Source: three-view drawing plus pictorial views. Frame: mm from the lowest corner of the part. Give positions to 0.01 mm unless a question says otherwise; leave off trailing zeros. Loops run counter-clockwise (first coordinate to the right, second up) from the corner with the lowest first, then second, coordinate; pieces in that order, holes last. Notation, with made-up numbers: M -36.5,-36.5 L -26.5,-36.5 A22 ccw -26.5,-7.5 Z; hole C 9.5,84 d2. An arc over 180 degrees is marked long. Answer as a JSON object with one key per item and string values. Group by question number.
1) Section query D-D on y = 14.25. Return loops of the section in (x, z), plus the area to 3 significant figures.
2) Section query A-A on y = 9.3. Return loops of the section in (x, z).
3) First-contact query: P1, Ø1.5, axis at x = 12, z = 4.5, coming from the -Y side; P2, Ø6, axis at y = 12.5, z = 10.5, coming from the +X side; P3, Ø4, axis at x = 2, z = 12, coming from the -Y side. Flat tips, straight axial feed; report the tip coordinate or a pass-through.
4) Draft query along Y for the marked faces 1, 2 and 3. Return one class per face: +Y half, -Y half, draft (parallel to the pull), parting line (faces both ways), or undercut.
5) Section query C-C on z = 11. Return loops of the section in (x, y), plus the area to 3 significant figures.
6) Ray query, L1, parallel to Y at x = 9.3, z = 7; L2, parallel to Y at x = 6, z = 11.5 (1 decimal); L3, parallel to X at y = 8.75, z = 8.75. Return the intervals inside material, ascending.
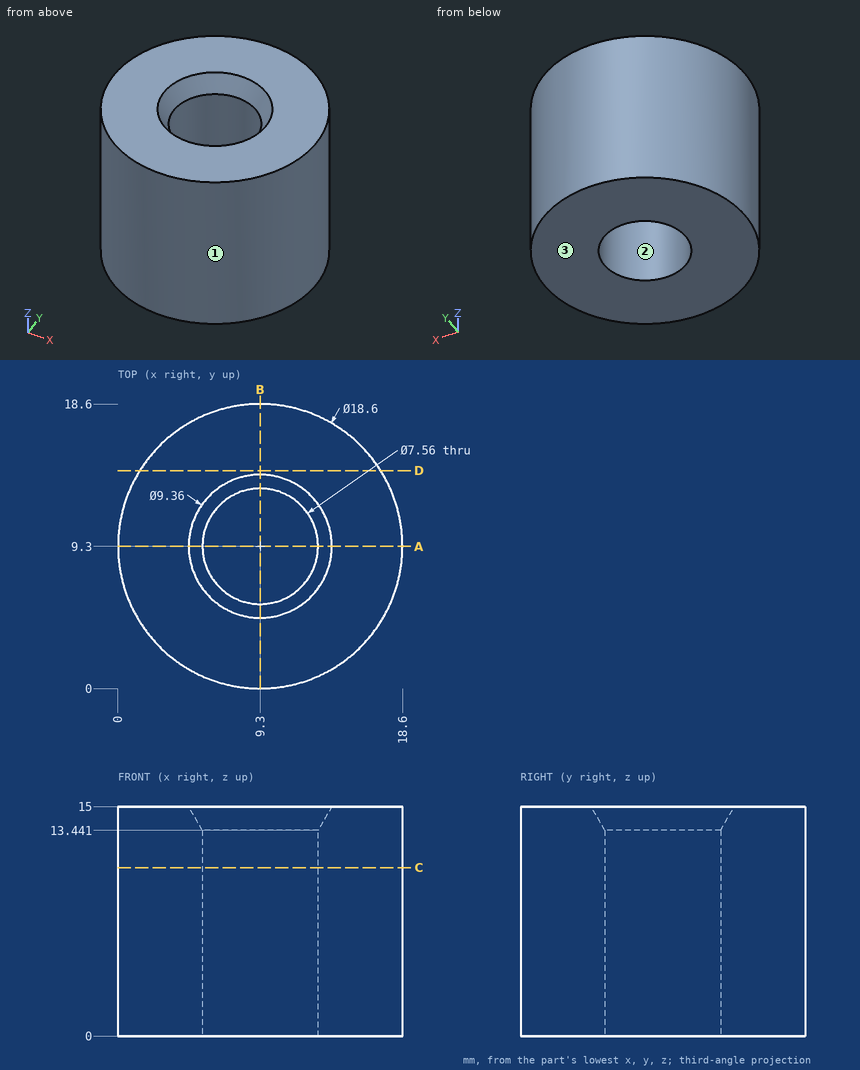
Output:
{
 "1": {"outline": "M 1.43,0 L 17.17,0 L 17.17,15 L 1.43,15 Z", "area": "236 mm^2"},
 "2": {"outline": "M 0,0 L 5.52,0 L 5.52,13.44 L 4.62,15 L 0,15 Z; M 13.08,0 L 18.6,0 L 18.6,15 L 13.98,15 L 13.08,13.44 Z"},
 "3": {"P1": "stops at y = 0.21", "P2": "stops at x = 18.6", "P3": "stops at y = 1.66"},
 "4": {"face 1": "parting line", "face 2": "undercut", "face 3": "draft"},
 "5": {"outline": "C 9.3,9.3 d18.6; hole C 9.3,9.3 d7.56", "area": "227 mm^2"},
 "6": {"L1": "y = 0 to 5.52, 13.08 to 18.6", "L2": "y = 0.6 to 7.5, 11.1 to 18", "L3": "x = 0.02 to 5.56, 13.04 to 18.58"}
}
